```python
from build123d import *

# Parameters (mm, degrees)
SKETCH_1_W          = 50
SKETCH_1_H          = 35
EXTRUDE_1_DEPTH     = 3
SKETCH_2_R          = 2.15
CUT_EXTRUDE_1_DEPTH = 3
SKETCH_3_R          = 2.15
CUT_EXTRUDE_2_DEPTH = 3
FILLET_1_R          = 3


with BuildPart() as part:
    # 草图1 → 凸台-拉伸1 (new body)
    with BuildSketch(Plane(origin=(0, 0, 0), x_dir=(1, 0, 0), z_dir=(0, 1, 0))):
        Rectangle(SKETCH_1_W, SKETCH_1_H)
    extrude(amount=EXTRUDE_1_DEPTH)

    # 草图2 → 切除-拉伸1 (cut)
    with BuildSketch(Plane(origin=(0, 3, 0), x_dir=(1, 0, 0), z_dir=(0, 1, 0))):
        with Locations((-15, 9.5)):
            Circle(SKETCH_2_R)
        with Locations((15, 9.5)):
            Circle(SKETCH_2_R)
    extrude(amount=-CUT_EXTRUDE_1_DEPTH, mode=Mode.SUBTRACT)

    # 草图3 → 切除-拉伸2 (cut)
    with BuildSketch(Plane(origin=(0, 3, 0), x_dir=(1, 0, 0), z_dir=(0, 1, 0))):
        with Locations((2, -7.5)):
            Circle(SKETCH_3_R)
        with Locations((10, -7.5)):
            Circle(SKETCH_3_R)
    extrude(amount=-CUT_EXTRUDE_2_DEPTH, mode=Mode.SUBTRACT)

    # 圆角1
    fillet_1_edges = [part.edges().sort_by_distance(p)[0] for p in [
        (25, 1.5, 17.5),
        (-25, 1.5, 17.5),
        (-25, 1.5, -17.5),
        (25, 1.5, -17.5),
    ]]
    fillet(fillet_1_edges, radius=FILLET_1_R)


solid = part.part
```
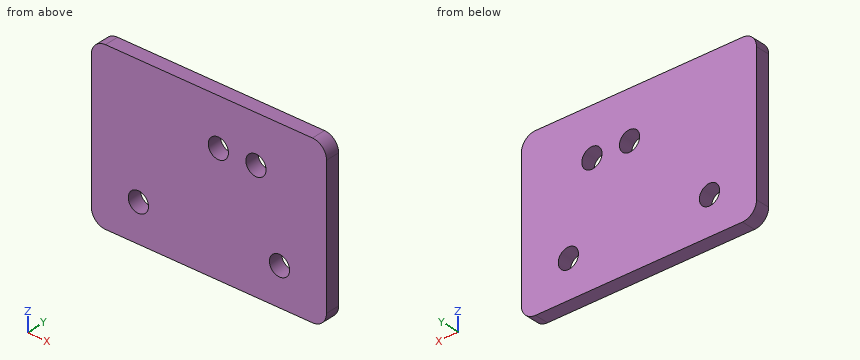
Part model, mm, in its own coordinate system. Round coordinates to 2 decimals unless told otherwise and drop trailing zeros. Loops run counter-clockwise (first coordinate to the right, second up) from the corner with the lowest first, then second, coordinate; pieces in that order, holes last. Notation, with made-up numbers: (46, 35.25) -> (88, 35.25) arc R11 ccw to (88, 52.25) -> close; hole circle Ø3 at (29, 38). An arc over 180 degrees is marked (long way). Use CSV: the item, a comma, the result in double quotes. Start each with the question number.
1) Cut at D-D, the plane z = -11. Write the cut outline in (x, y), plus the area to 3 significant figures.
2) Drop a flat-ended pin along its axis: P1, Ø4, axis at x = 2, z = 7.5, coming from the +Y side. Give the stop position or say it passes through.
3) Cut at A-A, the plane z = 7.5. Write the cut outline in (x, y).
4) Cut at C-C, the plane y = 2.55. Write the cut outline in (x, z), plus the area to 3 significant figures.
5) Cut at B-B, the plane x = 10. Write the cut outline in (y, z), plus the area to 3 significant figures.
6) Wall check: L1, parallel to X at y = 0.7, z = -9.5; L2, parallel to X at y = 2.2, z = 7.5; L3, parallel to Z at x = 15, y = 2.35. Give the ranges that are in metal, low to high. Write a range as [from, to].
Determined:
1,outline,"(-25, 0) -> (-16.54, 0) -> (-16.54, 3) -> (-25, 3) -> close; (-13.46, 0) -> (13.46, 0) -> (13.46, 3) -> (-13.46, 3) -> close; (16.54, 0) -> (25, 0) -> (25, 3) -> (16.54, 3) -> close"
1,area,"132 mm2"
2,P1,"passes through"
3,outline,"(-25, 0) -> (-0.15, 0) -> (-0.15, 3) -> (-25, 3) -> close; (4.15, 0) -> (7.85, 0) -> (7.85, 3) -> (4.15, 3) -> close; (12.15, 0) -> (25, 0) -> (25, 3) -> (12.15, 3) -> close"
4,outline,"(-25, -14.5) arc R3 ccw to (-22, -17.5) -> (22, -17.5) arc R3 ccw to (25, -14.5) -> (25, 14.5) arc R3 ccw to (22, 17.5) -> (-22, 17.5) arc R3 ccw to (-25, 14.5) -> close; hole circle Ø4.3 at (-15, -9.5); hole circle Ø4.3 at (2, 7.5); hole circle Ø4.3 at (10, 7.5); hole circle Ø4.3 at (15, -9.5)"
4,area,"1,680 mm2"
5,outline,"(0, -17.5) -> (3, -17.5) -> (3, 5.35) -> (0, 5.35) -> close; (0, 9.65) -> (3, 9.65) -> (3, 17.5) -> (0, 17.5) -> close"
5,area,"92.1 mm2"
6,L1,"x = [-25, -17.15], [-12.85, 12.85], [17.15, 25]"
6,L2,"x = [-25, -0.15], [4.15, 7.85], [12.15, 25]"
6,L3,"z = [-17.5, -11.65], [-7.35, 17.5]"
